from build123d import *

# Parameters (mm, degrees)
SKETCH1_R           = 7.5
BOSS_EXTRUDE1_DEPTH = 5
SKETCH3_2_W         = 140
SKETCH3_2_H         = 5
BOSS_EXTRUDE3_DEPTH = 35
FILLET1_R           = 2


with BuildPart() as part:
    # Sketch1 → Boss-Extrude1 (new body)
    with BuildSketch(Plane(origin=(0, 0, 0), x_dir=(0, 0, -1), z_dir=(1, 0, 0))):
        Polygon((0, 20), (-80, -10), (-80, -40), (60, -40), (60, -10), align=None)
        Circle(SKETCH1_R, mode=Mode.SUBTRACT)
    extrude(amount=BOSS_EXTRUDE1_DEPTH)

    # Sketch3<2> → Boss-Extrude3 (add)
    with BuildSketch(Plane(origin=(5, 0, 0), x_dir=(0, 0, -1), z_dir=(1, 0, 0))):
        with Locations((-10, -37.5)):
            Rectangle(SKETCH3_2_W, SKETCH3_2_H)
    extrude(amount=-BOSS_EXTRUDE3_DEPTH)

    # Fillet1
    fillet1_edges = [part.edges().sort_by_distance(p)[0] for p in [
        (-12.5, -40, -60),
        (-12.5, -40, 80),
    ]]
    fillet(fillet1_edges, radius=FILLET1_R)


solid = part.part
Here's how the part is built. I have some questions about the finished solid (model axes, mm). A direction names the side the tool comes from. Give positions to 0.01 mm unless a question says otherwise; leave off trailing zeros. Loops run counter-clockwise (first coordinate to the right, second up) from the corner with the lowest first, then second, coordinate; pieces in that order, holes last. Notation, with made-up numbers: (37, 33) -> (75, 33) arc R24 ccw to (75, 61) -> close; hole circle Ø5 at (25.5, -4). An arc over 180 degrees is marked (long way). Answer as a JSON object with one key per item and string values. Group by question number.
Item 1: Imagine slicing it at C-C on z = -44.5. Write out the boundary of the cut face in (x, y), then the cut area to 3 significant figures.
Item 2: Thinking about a two-plate mould opening in Z: for faces 1 (the flat face through (-30, -37, 11)), 2 (the cylindrical face through (2.465, 0.33, 7.493)), 3 (the flat face through (2, -29, 80)), which applies, pulls with the +Z half, pulls with the -Z half, needs draft (parallel to the pull), parting line crosses it, or undercut?
Item 3: On a 3-axis mill with a long thin cutter (end or side, diameter ignored), from which of +Z, -Z, +X, -X, +Y, -Y can I reach the whole of each face in a straight line? I mean faces 4 (the flat face through (2, 5, -30)), 5 (the flat face through (-15, -35, 11)). Say none if no direction works.
Item 4: Imagine slicing it at A-A on y = 0. Write out the boundary of the cut face in (x, z), then the cut area to 3 significant figures.
Item 5: Imagine slicing it at D-D on x = -4.5. Write out the boundary of the cut face in (y, z), then the cut area to 3 significant figures.
Item 6: Will these pins go through, and if not, where does the flat tip stop? pin 1 (24 mm diameter, centred on y = 0, z = 0, fed in from -X); pin 2 (2 mm diameter, centred on x = -16.5, z = 9, fed in from +Y); pin 3 (8 mm diameter, centred on x = -3, z = -32.5, fed in from +Y).
Item 7: I need wall thicknesses on L1, parallel to X at y = -13.5, z = 62.5; L2, parallel to Y at x = 3, z = 0; L3, parallel to Y at x = -17.5, z = -47.5. Which ranges of each line are inside material? Lowest first, please.
Item 8: Imagine slicing it at B-B on x = 2.5. Write out the boundary of the cut face in (y, z), then the cut area to 3 significant figures.
Answer list:
{
 "1": {"outline": "(-30, -40) -> (5, -40) -> (5, -2.25) -> (0, -2.25) -> (0, -35) -> (-30, -35) -> close", "area": "339 mm2"},
 "2": {"face 1": "needs draft", "face 2": "undercut", "face 3": "pulls with the +Z half"},
 "3": {"face 4": "-Z, +X, -X, +Y", "face 5": "+Z, -Z, -X, +Y"},
 "4": {"outline": "(0, -40) -> (5, -40) -> (5, -7.5) -> (0, -7.5) -> close; (0, 7.5) -> (5, 7.5) -> (5, 53.33) -> (0, 53.33) -> close", "area": "392 mm2"},
 "5": {"outline": "(-40, -58) arc R2 ccw to (-38, -60) -> (-35, -60) -> (-35, 80) -> (-38, 80) arc R2 ccw to (-40, 78) -> close", "area": "698 mm2"},
 "6": {"pin 1": "stops at x = 0", "pin 2": "stops at y = -35", "pin 3": "stops at y = 5.07"},
 "7": {"L1": "x = 0 to 5", "L2": "y = -40 to -7.5, 7.5 to 20", "L3": "y = -40 to -35"},
 "8": {"outline": "(-40, -58) arc R2 ccw to (-38, -60) -> (-10, -60) -> (20, 0) -> (-10, 80) -> (-38, 80) arc R2 ccw to (-40, 78) -> close; hole circle Ø15 at (0, 0)", "area": "6,120 mm2"}
}
